Autodesk Inventor part; units mm, degrees
ref_plane "Work Plane2" through (0, 76.2, 0) normal (0, 1, 0) x (-1, 0, 0)
ref_plane "YZ Plane" through (0, 0, 0) normal (1, 0, 0) x (0, 1, 0)
ref_plane "XY Plane" through (0, 0, 0) normal (0, 0, 1) x (1, 0, 0)
sketch "Sketch1" plane through (0, 0, 0) normal (0, 0, 1) x (1, 0, 0)
  circle A0 centre (0, 0) radius 76.2
  dimension "d0" = 152.4
extrude "Extrusion1" add sketch "Sketch1" along normal mid plane 2438.4
ref_plane "Work Plane2" through (0, 76.2, 0) normal (0, 1, 0) x (-1, 0, 0)
sketch "Sketch4" plane through (0, 76.2, 0) normal (0, 1, 0) x (-1, 0, 0)
  line L0 (25.4, 635) -> (25.4, 584.2)
  line L1 (25.4, 584.2) -> (-25.4, 584.2)
  line L2 (-25.4, 584.2) -> (-25.4, 635)
  line L3 (-25.4, 635) -> (25.4, 635)
  line L4 (25.4, 635) -> (-25.4, 584.2) construction
  line L5 (25.4, 584.2) -> (-25.4, 635) construction
  line L6 (76.2, 1219.2) -> (-76.2, 1219.2)
  point P0 (0, 0)
  point P1 (0, 609.6)
  dimension "d17" = 50.8
  dimension "d19" = 609.6
extrude "Extrusion3" add sketch "Sketch4" against normal blind 25.4
mirror "Mirror1" about plane through (0, 0, 0) normal (0, 0, 1) of "Extrusion3"
sketch "Sketch5" plane through (0, 76.2, 0) normal (0, 1, 0) x (1, 0, 0)
  line L0 (76.2, 1219.2) -> (-76.2, 1219.2)
  line L1 (-76.2, -1219.2) -> (76.2, -1219.2)
  point P0 (0, 0)
  point P1 (0, -609.6)
  point P2 (0, 609.6)
  dimension "d22" = 609.6
  dimension "d23" = 609.6
hole "Hole2" at (0, 76.2, 609.6) at (0, 76.2, -609.6) direction (0, -1, 0) diameter 25.4 end through all
properties part number "CrossMember-6-Feet" material "Wood (Walnut)"
Verification items for the finished model (mm, model axes). Coordinates: 2 decimals unless noted, no trailing zeros. Loops run counter-clockwise (first coordinate to the right, second up) from the corner with the lowest first, then second, coordinate; pieces in that order, holes last. Notation, with made-up numbers: (84, 66.25) -> (107, 66.25) arc R14 cw to (107, 77.25) -> close; hole circle Ø9 at (84.25, 84). An arc over 180 degrees is marked (long way). Answer in a Markdown table with one row per item. Add a question column.
1. Material ranges on probe 1 along Z at (x, y) = (0, 36.5); probe 2 along X at (y, z) = (1, 609.6); probe 3 along X at (y, z) = (-2, 612), recorded low to high. Write a range as [from, to].
2. Depth check by flat-ended pin: P1, Ø1, axis at y = 57.5, z = 585.5, coming from the -X side; P2, Ø2, axis at x = 13, z = 440.5, coming from the -Y side; P3, Ø20.5, axis at x = 0, z = 609.6, coming from the +Y side; P4, Ø1.3, axis at x = 18, y = 75, coming from the -Z side. Enter the tip coordinate at first touch or a pass-through.
3. Section check B-B, the plane y = -47. Enter the section's corners in (x, z), then the cut area to 3 significant figures.
4. Section check A-A, the plane z = -944. Enter the section's corners in (x, y), then the cut area to 3 significant figures.
5. Section check D-D, the plane x = 45. Enter the section's corners in (y, z), then the cut area to 3 significant figures.
6. Section check C-C, the plane x = -48. Enter the section's corners in (y, z).
Derived:
| question | item | result |
|---|---|---|
| 1 | probe 1 | z = [-1219.2, -622.3], [-596.9, 596.9], [622.3, 1219.2] |
| 1 | probe 2 | x = [-76.19, -12.7], [12.7, 76.19] |
| 1 | probe 3 | x = [-76.17, -12.47], [12.47, 76.17] |
| 2 | P1 | stops at x = -50.57 |
| 2 | P2 | stops at y = -75.25 |
| 2 | P3 | passes through |
| 2 | P4 | stops at z = -635 |
| 3 | outline | (-59.98, -1219.2) -> (59.98, -1219.2) -> (59.98, 1219.2) -> (-59.98, 1219.2) -> close; hole circle Ø25.4 at (0, -609.6); hole circle Ø25.4 at (0, 609.6) |
| 3 | area | 291,000 mm² |
| 4 | outline | circle Ø152.4 at (0, 0) |
| 4 | area | 18,200 mm² |
| 5 | outline | (-61.49, -1219.2) -> (61.49, -1219.2) -> (61.49, 1219.2) -> (-61.49, 1219.2) -> close |
| 5 | area | 300,000 mm² |
| 6 | outline | (-59.18, -1219.2) -> (59.18, -1219.2) -> (59.18, 1219.2) -> (-59.18, 1219.2) -> close |
